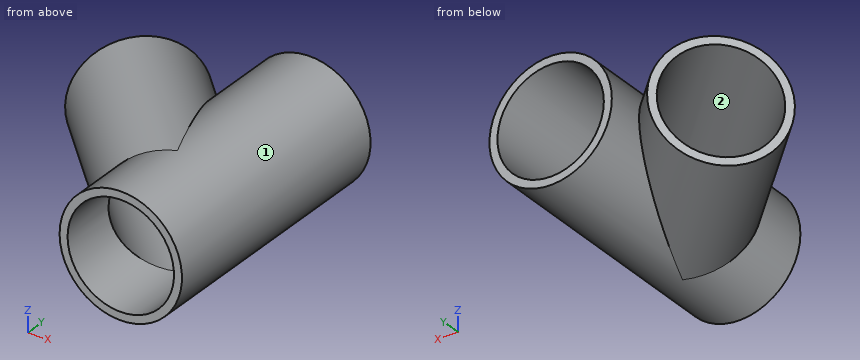
Autodesk Inventor part; units mm, degrees
ref_plane "Work Plane1" through (0, 0, 0) normal (-0.7071, 0.7071, 0) x (0, 0, 1)
ref_plane "YZ Plane" through (0, 0, 0) normal (1, 0, 0) x (0, 1, 0)
ref_plane "XY Plane" through (0, 0, 0) normal (0, 0, 1) x (1, 0, 0)
sketch "Sketch1" plane through (0, 0, 0) normal (0, 1, 0) x (-1, 0, 0)
  circle A0 centre (0, 0) radius 20
  circle A1 centre (0, 0) radius 23
  dimension "d0" = 40
  dimension "d1" = 46
extrude "Extrusion1" add sketch "Sketch1" along normal mid plane 140
ref_plane "Work Plane1" through (0, 0, 0) normal (-0.7071, 0.7071, 0) x (0, 0, 1)
sketch "Sketch2" plane through (0, 0, 0) normal (-0.7071, 0.7071, 0) x (0, 0, 1)
  circle A0 centre (0, 0) radius 20
  circle A1 centre (0, 0) radius 23
  dimension "d5" = 40
  dimension "d6" = 46
extrude "Extrusion2" add sketch "Sketch2" along normal blind 70
sketch "Sketch3" plane through (0, 70, 0) normal (0, 1, 0) x (1, 0, 0)
  circle A0 centre (0, 0) radius 20
extrude "Extrusion3" cut sketch "Sketch3" against normal through all
sketch "Sketch4" plane through (-49.4975, 49.4975, 0) normal (-0.7071, 0.7071, 0) x (-0.7071, -0.7071, 0)
  circle A0 centre (0, 0) radius 20
extrude "Extrusion4" cut sketch "Sketch4" against normal up to next
sketch "Sketch5" plane through (0, -70, 0) normal (0, -1, 0) x (1, 0, 0)
  circle A0 centre (0, 0) radius 20
  circle A1 centre (0, 0) radius 23
extrude "Extrusion5" cut sketch "Sketch5" against normal blind 40
properties part number "16217 - 40mm Plain PVC 45 Degree Tee" material "PVC-Piping"
CAD build for the part. Positions are in the model's coordinates, mm. Face numbers are marked on the shaded views. Coordinates: 2 decimals unless noted, no trailing zeros. Order: outer loops, then holes, each group sorted by start corner. A loop starts at its lowest first (then second) coordinate and runs counter-clockwise, first axis right, second up.
(1) Mould opens along Z. For the marked faces 1 and 2 say: released by +Z, released by -Z, zero draft, split by the parting line, or undercut.
Solution:
face 1: split by the parting line
face 2: undercut
(2) Saw through at D-D, the plane y = 57. Count the separate pieces of the cut face and the enclosed holes in it, and give its area (3 significant figures).
Solution:
separate pieces: 2
enclosed holes: 1
area: 598 mm2
(3) Saw through at C-C, the plane z = -11.5. Write the cut outline in (x, y).
Solution:
outline: (-63.58, 35.41) - (-19.92, -8.25) - (-19.92, -30) - (-16.36, -30) - (-16.36, -6.78) - (-61.07, 37.93) - close; (-37.93, 61.07) - (-16.36, 39.5) - (-16.36, 70) - (-19.92, 70) - (-19.92, 48.09) - (-35.41, 63.58) - close; (16.36, -30) - (19.92, -30) - (19.92, 70) - (16.36, 70) - close
(4) Pin check, flat tips, straight feed: pin 1 Ø3 at (x, y) = (7, 52) entering from -Z; pin 2 Ø12 at (x, z) = (-51, -6.5) entering from +Y; pin 3 Ø6 at (x, y) = (-21.5, -10) entering from -Z. Stop position of each tip, or through.
Solution:
pin 1: stops at z = -22.33
pin 2: stops at y = 31.4
pin 3: stops at z = -13.67
(5) Drill centre lines: L1, parallel to Z at x = 0, y = 47; L2, parallel to X at y = 65, z = 8; L3, parallel to Z at x = -30, y = 3.5. Where is each one in solid material? Low to high.
Solution:
L1: z = -23 to -20, 20 to 23
L2: x = -21.56 to -18.33, 18.33 to 21.56
L3: z = -13.34 to -6.99, 6.99 to 13.34
(6) Saw through at B-B, the plane x = 17. Write the cut outline in (y, z), and give its area (3 significant figures).
Solution:
outline: (-30, -15.49) - (70, -15.49) - (70, -10.54) - (-30, -10.54) - close; (-30, 10.54) - (70, 10.54) - (70, 15.49) - (-30, 15.49) - close
area: 991 mm2
(7) Saw through at A-A, the plane z = 0. Write the cut outline in (x, y), and give its area (3 significant figures).
Solution:
outline: (-65.76, 33.23) - (-23, -9.53) - (-23, -30) - (-20, -30) - (-20, -8.28) - (-63.64, 35.36) - close; (-35.36, 63.64) - (-20, 48.28) - (-20, 70) - (-23, 70) - (-23, 55.53) - (-33.23, 65.76) - close; (20, -30) - (23, -30) - (23, 70) - (20, 70) - close
area: 655 mm2
